Job drawing, mm, ordinate dimensions from the low corner. One solid piece. A direction names the side the tool comes from. Round coordinates to 2 decimals unless told otherwise and drop trailing zeros. Loops run counter-clockwise (first coordinate to the right, second up) from the corner with the lowest first, then second, coordinate; pieces in that order, holes last.
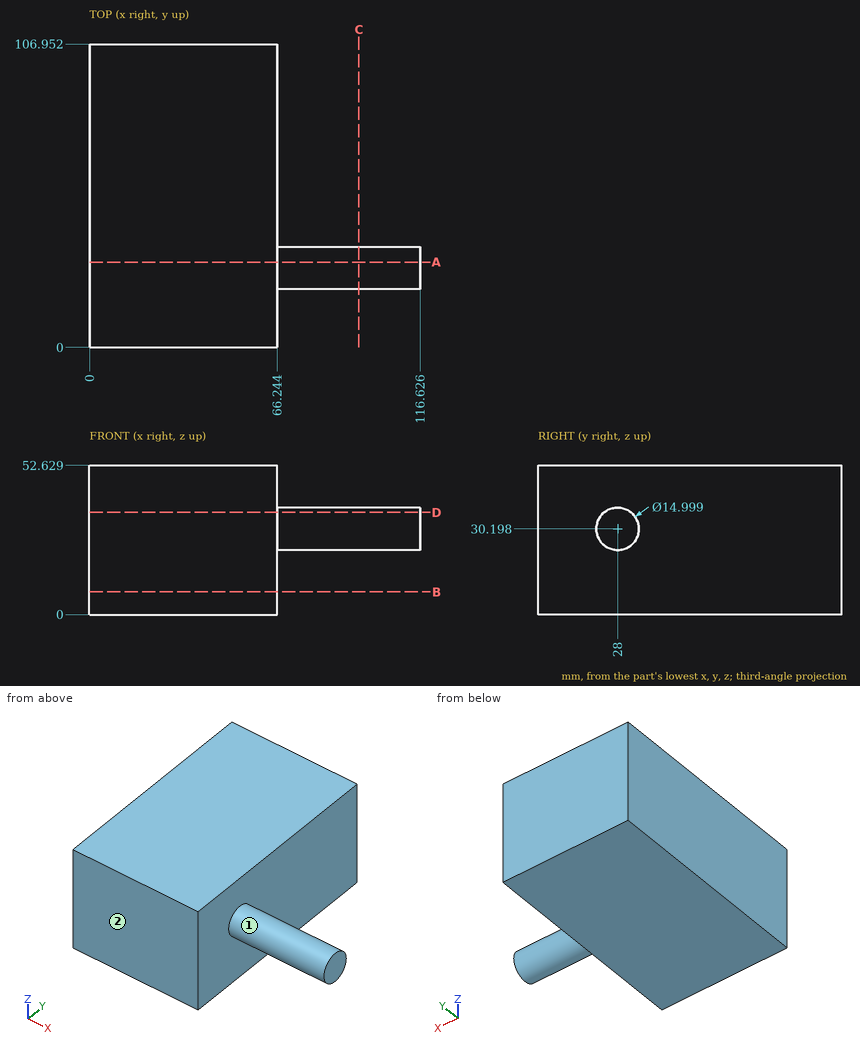
1) Slice it at D-D, the plane z = 36. Give the cut face in (x, y), then the cut area to 3 significant figures.
Values:
outline: (0, 0) - (66.24, 0) - (66.24, 23.25) - (116.63, 23.25) - (116.63, 32.75) - (66.24, 32.75) - (66.24, 106.95) - (0, 106.95) - close
area: 7,560 mm2
2) Tool access for the marked faces 1 and 2: list every direction of +Z, -Z, +X, -X, +Y, -Y with a clear straight run to the whole face (end or side of a thin tool).
Values:
face 1: +X
face 2: +Z, -Z, +X, -X, -Y
3) Wall check: line 1 along X through (y, z) = (30.5, 19.5); line 2 along Y through (x, z) = (77, 30.5). Give the ranges that are in metal, low to high.
Values:
line 1: x = 0 to 66.24
line 2: y = 20.51 to 35.49
4) Drop flat-ended pins along their axis: pin 1 Ø4 at (x, z) = (103, 28.5) entering from +Y; pin 2 Ø1.5 at (x, z) = (85.5, 25) entering from -Y; pin 3 Ø4 at (y, z) = (73, 10.5) entering from +X. Give the stop position or say it passes through.
Values:
pin 1: stops at y = 35.5
pin 2: stops at y = 21.96
pin 3: stops at x = 66.24
5) Slice it at B-B, the plane z = 8. Give the cut face in (x, y).
Values:
outline: (0, 0) - (66.24, 0) - (66.24, 106.95) - (0, 106.95) - close
6) Slice it at C-C, the plane x = 95. Give the cut face in (y, z).
Values:
outline: circle Ø15 at (28, 30.2)
7) Slice it at A-A, the plane y = 30. Give the cut face in (x, z), then the cut area to 3 significant figures.
Values:
outline: (0, 0) - (66.24, 0) - (66.24, 22.97) - (116.63, 22.97) - (116.63, 37.43) - (66.24, 37.43) - (66.24, 52.63) - (0, 52.63) - close
area: 4,210 mm2
